Can you work these out from the drawing? Everything is in mm from the part's minimum corner. Give positions to 0.01 mm unless a question says otherwise; leave off trailing zeros. Order: outer loops, then holes, each group sorted by start corner. A loop starts at its lowest first (then second) coordinate and runs counter-clockwise, first axis right, second up. Notation, with made-up numbers: (-16, -4) -> (33, -4) arc R20 ccw to (33, 3) -> close; hole circle Ø10 at (-33.75, 53.25). An arc over 180 degrees is marked (long way). One line per item, written item: value.
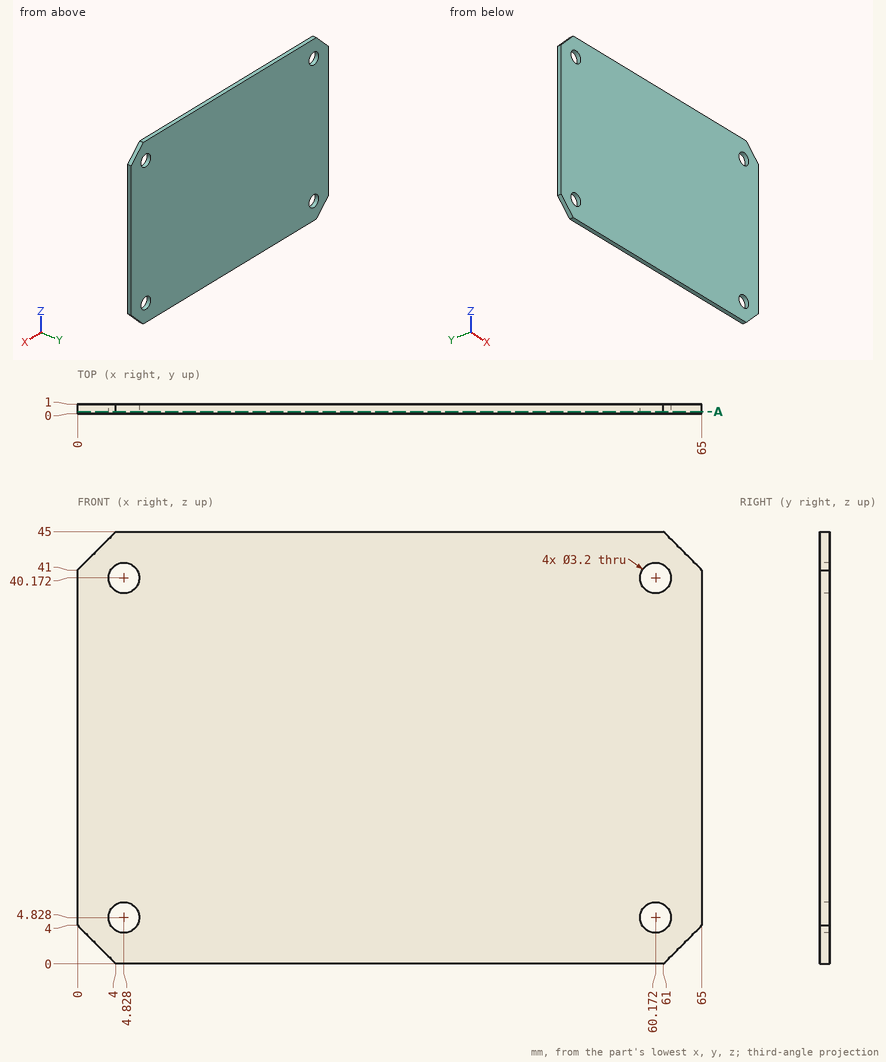
1) Suppose I cut it at A-A, the plane y = 0.2. Write out the boundary of the cut face in (x, z), then the cut area to 3 significant figures.
Answer below:
outline: (0, 4) -> (4, 0) -> (61, 0) -> (65, 4) -> (65, 41) -> (61, 45) -> (4, 45) -> (0, 41) -> close; hole circle Ø3.2 at (4.83, 4.83); hole circle Ø3.2 at (4.83, 40.17); hole circle Ø3.2 at (60.17, 4.83); hole circle Ø3.2 at (60.17, 40.17)
area: 2,860 mm2
2) For P1, Ø3, axis at x = 60.17, z = 4.83, coming from the -Y side, with a flat end and sliding along its axis, tell me the tip position at first contact or that it passes through.
Answer below:
P1: passes through
3) If I drill on line 1 along X through (y, z) = (0.5, 40); line 2 along Z through (x, y) = (6, 0.35); line 3 along X through (y, z) = (0.7, 3.5) (1 decimal), over which ranges is the centre line in solid material (lowest first)?
Answer below:
line 1: x = 0 to 3.24, 6.42 to 58.58, 61.76 to 65
line 2: z = 0 to 3.74, 5.92 to 39.08, 41.26 to 45
line 3: x = 0.5 to 3.9, 5.7 to 59.3, 61.1 to 64.5
